Part model, mm, in its own coordinate system. Give positions to 0.01 mm unless a question says otherwise; leave off trailing zeros. Order: outer loops, then holes, each group sorted by start corner. A loop starts at its lowest first (then second) coordinate and runs counter-clockwise, first axis right, second up. Notation, with made-up numbers: M 82,70.25 L 103,70.25 A22 ccw 103,107.25 Z; hole C 8.25,45.25 d11. An arc over 180 degrees is marked long. Return JSON: item names as keys, results as strings.
from build123d import *

# Parameters (mm, degrees)
BOSS_EXTRUDE1_DEPTH       = 1.6
CUT_EXTRUDE3_REACH        = 3.6
SKETCH3_R                 = 1.55
SKETCH3_R_2               = 1.2
CUT_EXTRUDE4_REACH        = 3.6
PRESS_FIT_NUT_LOCATIONS_R = 2.78


with BuildPart() as part:
    # Outline → Boss-Extrude1 (new body)
    with BuildSketch(Plane.XY):
        with BuildLine():
            Line((-38.9, 21.1), (-38.9, -32.9))
            ThreePointArc((-38.9, -32.9), (-36.556854249, -38.556854249), (-30.9, -40.9))
            Line((-30.9, -40.9), (29.1, -40.9))
            ThreePointArc((29.1, -40.9), (37.585281374, -37.385281374), (41.1, -28.9))
            Line((41.1, -28.9), (41.1, 29.1))
            ThreePointArc((41.1, 29.1), (39.928427125, 31.928427125), (37.1, 33.1))
            Line((37.1, 33.1), (-26.9, 33.1))
            ThreePointArc((-26.9, 33.1), (-35.385281374, 29.585281374), (-38.9, 21.1))
        make_face()
    extrude(amount=BOSS_EXTRUDE1_DEPTH)

    # Sketch3 → Cut-Extrude3 (cut, up to next)
    with BuildSketch(Plane.XY.offset(1.6), mode=Mode.PRIVATE) as cut_extrude3_sk1:
        with Locations((-6.677e-06, 25.099991446)):
            Circle(SKETCH3_R)
    cut_extrude3_tool1 = extrude(cut_extrude3_sk1.sketch, amount=-CUT_EXTRUDE3_REACH, mode=Mode.PRIVATE) & part.part
    add(cut_extrude3_tool1.solids().sort_by_distance((-7e-06, 25.099991, 1.6))[0], mode=Mode.SUBTRACT)
    # Sketch3 → Cut-Extrude3 (cut, up to next)
    with BuildSketch(Plane.XY.offset(1.6), mode=Mode.PRIVATE) as cut_extrude3_sk2:
        with Locations((25.099993323, -8.554e-06)):
            Circle(SKETCH3_R_2)
    cut_extrude3_tool2 = extrude(cut_extrude3_sk2.sketch, amount=-CUT_EXTRUDE3_REACH, mode=Mode.PRIVATE) & part.part
    add(cut_extrude3_tool2.solids().sort_by_distance((25.099993, -9e-06, 1.6))[0], mode=Mode.SUBTRACT)
    # Sketch3 → Cut-Extrude3 (cut, up to next)
    with BuildSketch(Plane.XY.offset(1.6), mode=Mode.PRIVATE) as cut_extrude3_sk3:
        with Locations((-6.677e-06, -25.100008554)):
            Circle(SKETCH3_R)
    cut_extrude3_tool3 = extrude(cut_extrude3_sk3.sketch, amount=-CUT_EXTRUDE3_REACH, mode=Mode.PRIVATE) & part.part
    add(cut_extrude3_tool3.solids().sort_by_distance((-7e-06, -25.100009, 1.6))[0], mode=Mode.SUBTRACT)
    # Sketch3 → Cut-Extrude3 (cut, up to next)
    with BuildSketch(Plane.XY.offset(1.6), mode=Mode.PRIVATE) as cut_extrude3_sk4:
        with Locations((-25.100006677, -8.554e-06)):
            Circle(SKETCH3_R_2)
    cut_extrude3_tool4 = extrude(cut_extrude3_sk4.sketch, amount=-CUT_EXTRUDE3_REACH, mode=Mode.PRIVATE) & part.part
    add(cut_extrude3_tool4.solids().sort_by_distance((-25.100007, -9e-06, 1.6))[0], mode=Mode.SUBTRACT)

    # Press Fit Nut Locations → Cut-Extrude4 (cut, up to next)
    with BuildSketch(Plane.XY.offset(1.6), mode=Mode.PRIVATE) as cut_extrude4_sk1:
        with Locations((-27.030733336, 27.030733336)):
            Circle(PRESS_FIT_NUT_LOCATIONS_R)
    cut_extrude4_tool1 = extrude(cut_extrude4_sk1.sketch, amount=-CUT_EXTRUDE4_REACH, mode=Mode.PRIVATE) & part.part
    add(cut_extrude4_tool1.solids().sort_by_distance((-27.030733, 27.030733, 1.6))[0], mode=Mode.SUBTRACT)
    # Press Fit Nut Locations → Cut-Extrude4 (cut, up to next)
    with BuildSketch(Plane.XY.offset(1.6), mode=Mode.PRIVATE) as cut_extrude4_sk2:
        with Locations((27.030733336, 27.030733336)):
            Circle(PRESS_FIT_NUT_LOCATIONS_R)
    cut_extrude4_tool2 = extrude(cut_extrude4_sk2.sketch, amount=-CUT_EXTRUDE4_REACH, mode=Mode.PRIVATE) & part.part
    add(cut_extrude4_tool2.solids().sort_by_distance((27.030733, 27.030733, 1.6))[0], mode=Mode.SUBTRACT)
    # Press Fit Nut Locations → Cut-Extrude4 (cut, up to next)
    with BuildSketch(Plane.XY.offset(1.6), mode=Mode.PRIVATE) as cut_extrude4_sk3:
        with Locations((-27.030733336, -27.030733336)):
            Circle(PRESS_FIT_NUT_LOCATIONS_R)
    cut_extrude4_tool3 = extrude(cut_extrude4_sk3.sketch, amount=-CUT_EXTRUDE4_REACH, mode=Mode.PRIVATE) & part.part
    add(cut_extrude4_tool3.solids().sort_by_distance((-27.030733, -27.030733, 1.6))[0], mode=Mode.SUBTRACT)
    # Press Fit Nut Locations → Cut-Extrude4 (cut, up to next)
    with BuildSketch(Plane.XY.offset(1.6), mode=Mode.PRIVATE) as cut_extrude4_sk4:
        with Locations((27.030733336, -27.030733336)):
            Circle(PRESS_FIT_NUT_LOCATIONS_R)
    cut_extrude4_tool4 = extrude(cut_extrude4_sk4.sketch, amount=-CUT_EXTRUDE4_REACH, mode=Mode.PRIVATE) & part.part
    add(cut_extrude4_tool4.solids().sort_by_distance((27.030733, -27.030733, 1.6))[0], mode=Mode.SUBTRACT)


solid = part.part
Q1. Band-saw the part on A-A (x = -28). Give the cut face in (y, z), then the cut area to 3 significant figures.
Established:
{"outline": "M -40.9,0 L -29.64,0 L -29.64,1.6 L -40.9,1.6 Z; M -24.43,0 L 24.43,0 L 24.43,1.6 L -24.43,1.6 Z; M 29.64,0 L 33.05,0 L 33.05,1.6 L 29.64,1.6 Z", "area": "102 mm²"}
Q2. Pin check, flat tip, straight feed: pin 1 (9 mm diameter, centred on x = -27.03, y = -27.03, fed in from +Z). Stop position of the tip, or through.
Established:
{"pin 1": "stops at z = 1.6"}
Q3. Band-saw the part on B-B (z = 1.2). Give the number of separate pieces and of enclosed holes in the cut face, then the cut area to 3 significant figures.
Established:
{"separate pieces": "1", "enclosed holes": "8", "area": "5,720 mm²"}
Q4. Two-plate mould, pull along Y, no slides. Class faces 1 (the cylindrical face through (24.15, -0.73, 0.81)), 2 (the cylindrical face through (37.49, -37.48, 0.79)), 3 (the cylindrical face through (24.982, -25.152, 0.811)), 4 (the cylindrical face through (-35.29, 29.68, 0.79)): +Y half, -Y half, draft (parallel to the pull), parting line (faces both ways), or undercut.
Established:
{"face 1": "undercut", "face 2": "-Y half", "face 3": "undercut", "face 4": "+Y half"}
Q5. Probe line 1 along Y through (x, z) = (27, 0.9); line 2 along X through (y, z) = (25.5, 1.25); line 3 along X through (y, z) = (-29, 1.2). List the from-to ranges inside material, lowest first.
Established:
{"line 1": "y = -40.9 to -29.81, -24.25 to 24.25, 29.81 to 33.1", "line 2": "x = -38.06 to -29.35, -24.71 to -1.5, 1.5 to 24.71, 29.35 to 41.1", "line 3": "x = -38.9 to -28.99, -25.07 to 25.07, 28.99 to 41.1"}
